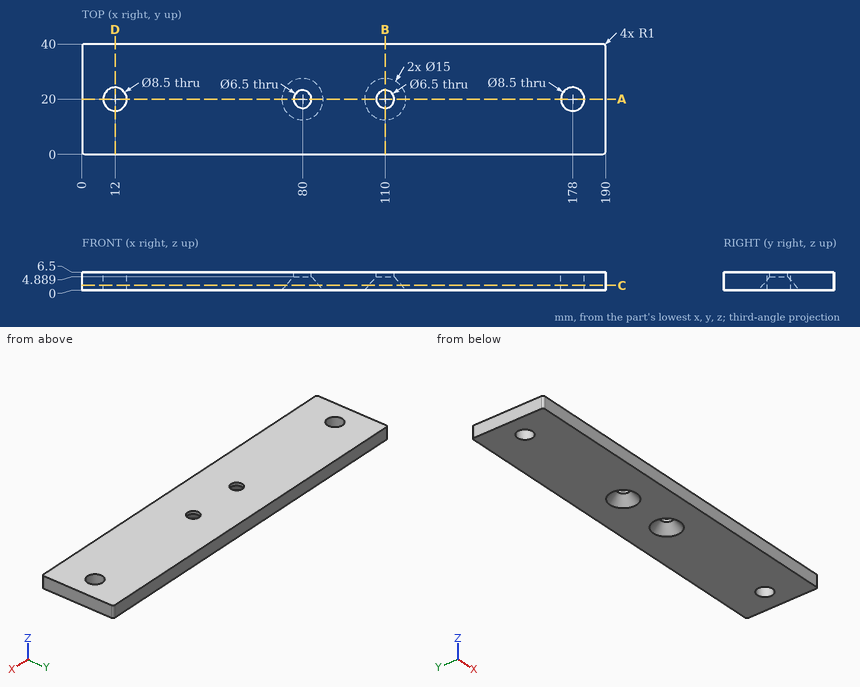
Job drawing, mm, ordinate dimensions from the low corner. One solid piece. Give positions to 0.01 mm unless a question says otherwise; leave off trailing zeros. Order: outer loops, then holes, each group sorted by start corner. A loop starts at its lowest first (then second) coordinate and runs counter-clockwise, first axis right, second up. Notation, with made-up numbers: (21, 55.25) -> (37, 55.25) arc R11 ccw to (37, 60.25) -> close; hole circle Ø10 at (49.25, -29.5). An arc over 180 degrees is marked (long way). Return JSON: item names as keys, results as strings.
Q1. Saw through at A-A (y = 20). Write the cut outline in (x, z), then the cut area to 3 significant figures.
Working result:
{"outline": "(0, 0) -> (7.75, 0) -> (7.75, 6.5) -> (0, 6.5) -> close; (16.25, 0) -> (72.5, 0) -> (76.75, 4.89) -> (76.75, 6.5) -> (16.25, 6.5) -> close; (83.25, 4.89) -> (87.5, 0) -> (102.5, 0) -> (106.75, 4.89) -> (106.75, 6.5) -> (83.25, 6.5) -> close; (113.25, 4.89) -> (117.5, 0) -> (173.75, 0) -> (173.75, 6.5) -> (113.25, 6.5) -> close; (182.25, 0) -> (190, 0) -> (190, 6.5) -> (182.25, 6.5) -> close", "area": "998 mm²"}
Q2. Saw through at B-B (x = 110). Write the cut outline in (y, z).
Working result:
{"outline": "(0, 0) -> (12.5, 0) -> (16.75, 4.89) -> (16.75, 6.5) -> (0, 6.5) -> close; (23.25, 4.89) -> (27.5, 0) -> (40, 0) -> (40, 6.5) -> (23.25, 6.5) -> close"}
Q3. Saw through at D-D (x = 12). Write the cut outline in (y, z), then the cut area to 3 significant figures.
Working result:
{"outline": "(0, 0) -> (15.75, 0) -> (15.75, 6.5) -> (0, 6.5) -> close; (24.25, 0) -> (40, 0) -> (40, 6.5) -> (24.25, 6.5) -> close", "area": "205 mm²"}
Q4. Flat gauge pin, fed straight in: pin 1 (7.5 mm diameter, centred on x = 110, y = 20, fed in from -Z). Where does the tip first touch, or does it go through?
Working result:
{"pin 1": "z = 4.31"}
Q5. Saw through at C-C (z = 1.75). Write the cut outline in (x, y).
Working result:
{"outline": "(0, 1) arc R1 ccw to (1, 0) -> (189, 0) arc R1 ccw to (190, 1) -> (190, 39) arc R1 ccw to (189, 40) -> (1, 40) arc R1 ccw to (0, 39) -> close; hole circle Ø8.5 at (12, 20); hole circle Ø11.96 at (80, 20); hole circle Ø11.96 at (110, 20); hole circle Ø8.5 at (178, 20)"}
Q6. Drill centre lines: line 1 (Y direction, x = 178, z = 2); line 2 (Y direction, x = 80, z = 6.05); line 3 (X direction, y = 23.5, z = 3). Where is each one in solid material? Low to high.
Working result:
{"line 1": "0 to 15.75, 24.25 to 40", "line 2": "0 to 16.75, 23.25 to 40", "line 3": "0 to 9.59, 14.41 to 76.58, 83.42 to 106.58, 113.42 to 175.59, 180.41 to 190"}
